from build123d import *

# Parameters (mm, degrees)
F0_W     = 125
F0_H     = 425
F1_DEPTH = 235
F2_R     = 15
F3_DEPTH = 15
F4_R     = 50
F5_DEPTH = 25


with BuildPart() as f1:
    # F0 (on Top) → F1 (new body)
    with BuildSketch(Plane.XY):
        Rectangle(F0_W, F0_H)
    extrude(amount=F1_DEPTH)

    # F2 (on face) → F3 (join)
    with BuildSketch(Plane.XZ.offset(212.5)):
        with Locations((-42.5, 20)):
            Circle(F2_R)
    extrude(amount=F3_DEPTH)

    # F4 (on face) → F5 (join)
    with BuildSketch(Plane.XY.offset(235)):
        with Locations((0, -152.5)):
            Circle(F4_R)
    extrude(amount=F5_DEPTH)


solid = f1.part
Geometry check sheet. Reference: the model listing, model coordinates, mm. A direction names the side the tool comes from. Round coordinates to 2 decimals unless told otherwise and drop trailing zeros. Write each loop counter-clockwise with the first axis right and the second up, starting at its lowest first coordinate (ties: lowest second). Pieces come first, ordered by that corner, then holes. Notation, with made-up numbers: (-8.5, 47.5) -> (7.5, 47.5) arc R21 ccw to (7.5, 70.5) -> close; hole circle Ø5 at (43.25, 57). An arc over 180 degrees is marked (long way). One line per item, written item: value. Start each with the question number.
(1) Cross-section at D-D, the plane z = 82.5. Record the cut outline in (x, y), and give its area (3 significant figures).
(2) Cross-section at C-C, the plane x = -36. Record the cut outline in (y, z), and give its area (3 significant figures).
(3) Cross-section at A-A, the plane y = -152.5. Record the cut outline in (x, z), and give its area (3 significant figures).
(4) Scan lines: line 1 (Y direction, x = 44.5, z = 144); line 2 (Z direction, x = -24.5, y = 58). Record each from-to range of solid material in increasing order. Write a range as [from, to].
(5) Cross-section at B-B, the plane z = 20. Record the cut outline in (x, y), and give its area (3 significant figures).
(6) Go/stop test with flat-tipped pins: pin 1 Ø1 at (x, y) = (-0.5, 110) entering from +Z; pin 2 Ø1 at (x, z) = (-26.5, 225) entering from -Y; pin 3 Ø5 at (x, y) = (33.5, -121) entering from -Z. Record where each tip stops, or that it passes through.
(7) Access from +Z, -Z, +X, -X, +Y, -Y to the whole of each face (thin tool, end or side, straight path). Record for faces 1 (the cylindrical face through (-54.4, -219.9, 10.87)), 2 (the cylindrical face through (47.69, -137.48, 247.32)), 3 (the flat face through (62.5, -3, 116)).
Answer:
1. outline: (-62.5, -212.5) -> (62.5, -212.5) -> (62.5, 212.5) -> (-62.5, 212.5) -> close
1. area: 53,100 mm²
2. outline: (-227.5, 6.48) -> (-212.5, 6.48) -> (-212.5, 0) -> (212.5, 0) -> (212.5, 235) -> (-117.8, 235) -> (-117.8, 260) -> (-187.2, 260) -> (-187.2, 235) -> (-212.5, 235) -> (-212.5, 33.52) -> (-227.5, 33.52) -> close
2. area: 102,000 mm²
3. outline: (-62.5, 0) -> (62.5, 0) -> (62.5, 235) -> (50, 235) -> (50, 260) -> (-50, 260) -> (-50, 235) -> (-62.5, 235) -> close
3. area: 31,900 mm²
4. line 1: [-212.5, 212.5]
4. line 2: [0, 235]
5. outline: (-62.5, -212.5) -> (-57.5, -212.5) -> (-57.5, -227.5) -> (-27.5, -227.5) -> (-27.5, -212.5) -> (62.5, -212.5) -> (62.5, 212.5) -> (-62.5, 212.5) -> close
5. area: 53,600 mm²
6. pin 1: z = 235
6. pin 2: y = -212.5
6. pin 3: z = 0
7. face 1: -Y
7. face 2: +Z
7. face 3: +Z, -Z, +X, +Y, -Y
